from build123d import *

# Parameters (mm, degrees)
BOSS_EXTRUDE1_DEPTH = 7.62
FILLET1_R           = 0.635


with BuildPart() as part:
    # Sketch1 → Boss-Extrude1 (new body)
    with BuildSketch(Plane.XY):
        Polygon((0, 0), (0, 12.7), (10.363, 12.7), (10.363, 1.575), (8.763, 1.575), (8.763, 11.1), (3.175, 11.1), (3.175, 0), align=None)
    extrude(amount=BOSS_EXTRUDE1_DEPTH)

    # Fillet1
    fillet1_edges = [part.edges().sort_by_distance(p)[0] for p in [
        (0, 0, 3.81),
        (0, 12.7, 3.81),
        (10.363, 12.7, 3.81),
        (10.363, 1.575, 3.81),
        (8.763, 1.575, 3.81),
        (8.763, 11.1, 3.81),
        (3.175, 11.1, 3.81),
        (3.175, 0, 3.81),
    ]]
    fillet(fillet1_edges, radius=FILLET1_R)


solid = part.part
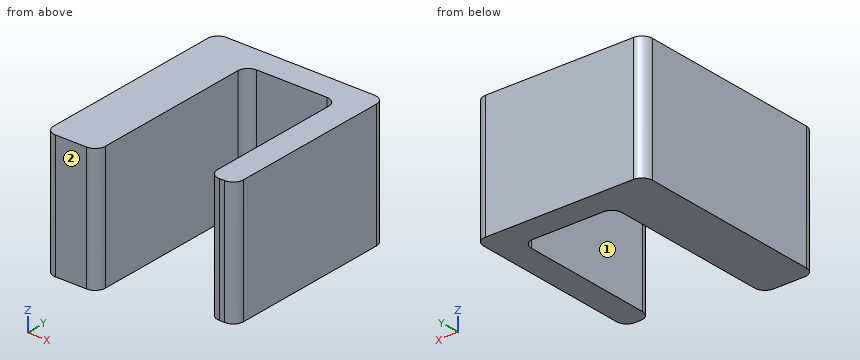
Geometry: final body of the model. Coordinates: model frame, mm. Face numbers are marked on the shaded views. A direction names the side the tool comes from. Coordinates: 2 decimals unless noted, no trailing zeros. Order: outer loops, then holes, each group sorted by start corner. A loop starts at its lowest first (then second) coordinate and runs counter-clockwise, first axis right, second up.
(1) Access query for the marked faces 1 and 2. Directions: +Z, -Z, +X, -X, +Y, -Y. A direction counts if a zero-diameter tool reaches every point of the face in a straight line with its end or side. Return the directions, or none.
(2) Material intervals for probe 1 along X at (y, z) = (2.75, 0.75) (3 decimals); probe 2 along Y at (x, z) = (5.75, 1.5); probe 3 along Y at (x, z) = (0.5, 2.5), sorted ascending.
(3) First-contact query: pin 1 (2 mm diameter, centred on x = 5.5, z = 2.5, fed in from -Y); pin 2 (1 mm diameter, centred on x = 5.5, y = 7, fed in from +Z). Flat tips, straight axial feed; report the tip coordinate or a pass-through.
(4) Section query B-B (z = 2.5). Return the cut outline in (x, y) (3 decimals).
(5) Section query C-C (x = 7). Return the cut outline in (y, z), plus the area to 3 significant figures.
(6) Section query A-A (y = 8.25). Return the cut outline in (x, z) (3 decimals), plus the area to 3 significant figures.
Solution:
1. face 1: +Z, -Z, -Y
1. face 2: +Z, -Z, +X, -X, -Y
2. probe 1: x = 0 to 3.175, 8.763 to 10.363
2. probe 2: y = 11.1 to 12.7
2. probe 3: y = 0.01 to 12.69
3. pin 1: stops at y = 11.1
3. pin 2: passes through
4. outline: (0, 0.635) arc R0.635 ccw to (0.635, 0) - (2.54, 0) arc R0.635 ccw to (3.175, 0.635) - (3.175, 10.465) arc R0.635 cw to (3.81, 11.1) - (8.128, 11.1) arc R0.635 cw to (8.763, 10.465) - (8.763, 2.21) arc R0.635 ccw to (9.398, 1.575) - (9.728, 1.575) arc R0.635 ccw to (10.363, 2.21) - (10.363, 12.065) arc R0.635 ccw to (9.728, 12.7) - (0.635, 12.7) arc R0.635 ccw to (0, 12.065) - close
5. outline: (11.1, 0) - (12.7, 0) - (12.7, 7.62) - (11.1, 7.62) - close
5. area: 12.2 mm2
6. outline: (0, 0) - (3.175, 0) - (3.175, 7.62) - (0, 7.62) - close; (8.763, 0) - (10.363, 0) - (10.363, 7.62) - (8.763, 7.62) - close
6. area: 36.4 mm2
